```python
from build123d import *

# Parameters (mm, degrees)
F0_R      = 2
F1_DEPTH  = 100
F1_FACE_R = 2
F2_DEPTH  = 140


with BuildPart() as f1:
    # F0 (on Front) → F1 (new body)
    with BuildSketch(Plane.XZ):
        with BuildLine():
            Line((8, -2), (8, 0))
            Line((8, 0), (8, 2))
            Line((8, 2), (10, 2))
            ThreePointArc((10, 2), (10.086846, 1.501846), (10.148892, 1))
            Line((10.148892, 1), (12.459936, 1))
            ThreePointArc((12.459936, 1), (11.548494, 4.783543), (9.517612, 8.103398))
            Line((9.517612, 8.103398), (7.883457, 6.469243))
            ThreePointArc((7.883457, 6.469243), (8.194443, 6.070511), (8.485281, 5.656854))
            Line((8.485281, 5.656854), (7.071068, 4.242641))
            Line((7.071068, 4.242641), (5.656854, 5.656854))
            Line((5.656854, 5.656854), (4.242641, 7.071068))
            Line((4.242641, 7.071068), (5.656854, 8.485281))
            ThreePointArc((5.656854, 8.485281), (6.070511, 8.194443), (6.469243, 7.883457))
            Line((6.469243, 7.883457), (8.103398, 9.517612))
            ThreePointArc((8.103398, 9.517612), (4.783543, 11.548494), (1, 12.459936))
            Line((1, 12.459936), (1, 10.148892))
            ThreePointArc((1, 10.148892), (1.501846, 10.086846), (2, 10))
            Line((2, 10), (2, 8))
            Line((2, 8), (0, 8))
            Line((0, 8), (-2, 8))
            Line((-2, 8), (-2, 10))
            ThreePointArc((-2, 10), (-1.501846, 10.086846), (-1, 10.148892))
            Line((-1, 10.148892), (-1, 12.459936))
            ThreePointArc((-1, 12.459936), (-4.783543, 11.548494), (-8.103398, 9.517612))
            Line((-8.103398, 9.517612), (-6.469243, 7.883457))
            ThreePointArc((-6.469243, 7.883457), (-6.070511, 8.194443), (-5.656854, 8.485281))
            Line((-5.656854, 8.485281), (-4.242641, 7.071068))
            Line((-4.242641, 7.071068), (-5.656854, 5.656854))
            Line((-5.656854, 5.656854), (-7.071068, 4.242641))
            Line((-7.071068, 4.242641), (-8.485281, 5.656854))
            ThreePointArc((-8.485281, 5.656854), (-8.194443, 6.070511), (-7.883457, 6.469243))
            Line((-7.883457, 6.469243), (-9.517612, 8.103398))
            ThreePointArc((-9.517612, 8.103398), (-11.548494, 4.783543), (-12.459936, 1))
            Line((-12.459936, 1), (-10.148892, 1))
            ThreePointArc((-10.148892, 1), (-10.086846, 1.501846), (-10, 2))
            Line((-10, 2), (-8, 2))
            Line((-8, 2), (-8, 0))
            Line((-8, 0), (-8, -2))
            Line((-8, -2), (-10, -2))
            ThreePointArc((-10, -2), (-10.086846, -1.501846), (-10.148892, -1))
            Line((-10.148892, -1), (-12.459936, -1))
            ThreePointArc((-12.459936, -1), (-11.548494, -4.783543), (-9.517612, -8.103398))
            Line((-9.517612, -8.103398), (-7.883457, -6.469243))
            ThreePointArc((-7.883457, -6.469243), (-8.194443, -6.070511), (-8.485281, -5.656854))
            Line((-8.485281, -5.656854), (-7.071068, -4.242641))
            Line((-7.071068, -4.242641), (-5.656854, -5.656854))
            Line((-5.656854, -5.656854), (-4.242641, -7.071068))
            Line((-4.242641, -7.071068), (-5.656854, -8.485281))
            ThreePointArc((-5.656854, -8.485281), (-6.070511, -8.194443), (-6.469243, -7.883457))
            Line((-6.469243, -7.883457), (-8.103398, -9.517612))
            ThreePointArc((-8.103398, -9.517612), (-4.783543, -11.548494), (-1, -12.459936))
            Line((-1, -12.459936), (-1, -10.148892))
            ThreePointArc((-1, -10.148892), (-1.501846, -10.086846), (-2, -10))
            Line((-2, -10), (-2, -8))
            Line((-2, -8), (0, -8))
            Line((0, -8), (2, -8))
            Line((2, -8), (2, -10))
            ThreePointArc((2, -10), (1.501846, -10.086846), (1, -10.148892))
            Line((1, -10.148892), (1, -12.459936))
            ThreePointArc((1, -12.459936), (4.783543, -11.548494), (8.103398, -9.517612))
            Line((8.103398, -9.517612), (6.469243, -7.883457))
            ThreePointArc((6.469243, -7.883457), (6.070511, -8.194443), (5.656854, -8.485281))
            Line((5.656854, -8.485281), (4.242641, -7.071068))
            Line((4.242641, -7.071068), (5.656854, -5.656854))
            Line((5.656854, -5.656854), (7.071068, -4.242641))
            Line((7.071068, -4.242641), (8.485281, -5.656854))
            ThreePointArc((8.485281, -5.656854), (8.194443, -6.070511), (7.883457, -6.469243))
            Line((7.883457, -6.469243), (9.517612, -8.103398))
            ThreePointArc((9.517612, -8.103398), (11.548494, -4.783543), (12.459936, -1))
            Line((12.459936, -1), (10.148892, -1))
            ThreePointArc((10.148892, -1), (10.086846, -1.501846), (10, -2))
            Line((10, -2), (8, -2))
        make_face()
        Circle(F0_R, mode=Mode.SUBTRACT)
    extrude(amount=F1_DEPTH)

    # F1_face (on face) → F2 (join)
    with BuildSketch(Plane.XZ.offset(100)):
        with BuildLine():
            ThreePointArc((6.469243, -7.883457), (6.070511, -8.194443), (5.656854, -8.485281))
            Line((5.656854, -8.485281), (4.242641, -7.071068))
            Line((4.242641, -7.071068), (7.071068, -4.242641))
            Line((7.071068, -4.242641), (8.485281, -5.656854))
            ThreePointArc((8.485281, -5.656854), (8.194443, -6.070511), (7.883457, -6.469243))
            Line((7.883457, -6.469243), (9.517612, -8.103398))
            ThreePointArc((9.517612, -8.103398), (11.548494, -4.783543), (12.459936, -1))
            Line((12.459936, -1), (10.148892, -1))
            ThreePointArc((10.148892, -1), (10.086846, -1.501846), (10, -2))
            Line((10, -2), (8, -2))
            Line((8, -2), (8, 2))
            Line((8, 2), (10, 2))
            ThreePointArc((10, 2), (10.086846, 1.501846), (10.148892, 1))
            Line((10.148892, 1), (12.459936, 1))
            ThreePointArc((12.459936, 1), (11.548494, 4.783543), (9.517612, 8.103398))
            Line((9.517612, 8.103398), (7.883457, 6.469243))
            ThreePointArc((7.883457, 6.469243), (8.194443, 6.070511), (8.485281, 5.656854))
            Line((8.485281, 5.656854), (7.071068, 4.242641))
            Line((7.071068, 4.242641), (4.242641, 7.071068))
            Line((4.242641, 7.071068), (5.656854, 8.485281))
            ThreePointArc((5.656854, 8.485281), (6.070511, 8.194443), (6.469243, 7.883457))
            Line((6.469243, 7.883457), (8.103398, 9.517612))
            ThreePointArc((8.103398, 9.517612), (4.783543, 11.548494), (1, 12.459936))
            Line((1, 12.459936), (1, 10.148892))
            ThreePointArc((1, 10.148892), (1.501846, 10.086846), (2, 10))
            Line((2, 10), (2, 8))
            Line((2, 8), (-2, 8))
            Line((-2, 8), (-2, 10))
            ThreePointArc((-2, 10), (-1.501846, 10.086846), (-1, 10.148892))
            Line((-1, 10.148892), (-1, 12.459936))
            ThreePointArc((-1, 12.459936), (-4.783543, 11.548494), (-8.103398, 9.517612))
            Line((-8.103398, 9.517612), (-6.469243, 7.883457))
            ThreePointArc((-6.469243, 7.883457), (-6.070511, 8.194443), (-5.656854, 8.485281))
            Line((-5.656854, 8.485281), (-4.242641, 7.071068))
            Line((-4.242641, 7.071068), (-7.071068, 4.242641))
            Line((-7.071068, 4.242641), (-8.485281, 5.656854))
            ThreePointArc((-8.485281, 5.656854), (-8.194443, 6.070511), (-7.883457, 6.469243))
            Line((-7.883457, 6.469243), (-9.517612, 8.103398))
            ThreePointArc((-9.517612, 8.103398), (-11.548494, 4.783543), (-12.459936, 1))
            Line((-12.459936, 1), (-10.148892, 1))
            ThreePointArc((-10.148892, 1), (-10.086846, 1.501846), (-10, 2))
            Line((-10, 2), (-8, 2))
            Line((-8, 2), (-8, -2))
            Line((-8, -2), (-10, -2))
            ThreePointArc((-10, -2), (-10.086846, -1.501846), (-10.148892, -1))
            Line((-10.148892, -1), (-12.459936, -1))
            ThreePointArc((-12.459936, -1), (-11.548494, -4.783543), (-9.517612, -8.103398))
            Line((-9.517612, -8.103398), (-7.883457, -6.469243))
            ThreePointArc((-7.883457, -6.469243), (-8.194443, -6.070511), (-8.485281, -5.656854))
            Line((-8.485281, -5.656854), (-7.071068, -4.242641))
            Line((-7.071068, -4.242641), (-4.242641, -7.071068))
            Line((-4.242641, -7.071068), (-5.656854, -8.485281))
            ThreePointArc((-5.656854, -8.485281), (-6.070511, -8.194443), (-6.469243, -7.883457))
            Line((-6.469243, -7.883457), (-8.103398, -9.517612))
            ThreePointArc((-8.103398, -9.517612), (-4.783543, -11.548494), (-1, -12.459936))
            Line((-1, -12.459936), (-1, -10.148892))
            ThreePointArc((-1, -10.148892), (-1.501846, -10.086846), (-2, -10))
            Line((-2, -10), (-2, -8))
            Line((-2, -8), (2, -8))
            Line((2, -8), (2, -10))
            ThreePointArc((2, -10), (1.501846, -10.086846), (1, -10.148892))
            Line((1, -10.148892), (1, -12.459936))
            ThreePointArc((1, -12.459936), (4.783543, -11.548494), (8.103398, -9.517612))
            Line((8.103398, -9.517612), (6.469243, -7.883457))
        make_face()
        Circle(F1_FACE_R, mode=Mode.SUBTRACT)
    extrude(amount=F2_DEPTH)


solid = f1.part
```
For this review, take the finished solid that the model builds, in its own axes (mm). A direction names the side the tool comes from. Coordinates: 2 decimals unless noted, no trailing zeros. Put each result on its own line as item: value.
1. Mouldability with a two-part tool opening along Z and no side actions: class faces 1 (the cylindrical face through (0, -118, -2)), 2 (the flat face through (8, -118, 0)), 3 (the cylindrical face through (-11.53, -118.32, 4.83)), 4 (the cylindrical face through (4.73, -118.32, -11.57)) as released by +Z, released by -Z, zero draft, split by the parting line, or undercut.
Values found:
face 1: undercut
face 2: undercut
face 3: released by +Z
face 4: released by -Z
2. For pin 1 (0.6 mm diameter, centred on x = -9, y = -85.5, fed in from -Z); pin 2 (1.8 mm diameter, centred on y = -62.5, z = 11, fed in from +X); pin 3 (3 mm diameter, centred on x = 4, y = -87, fed in from +Z); pin 4 (2 mm diameter, centred on x = 6.5, z = 9, fed in from +Y), all flat-tipped, find the tip position at first contact; note any pin that passes through.
Values found:
pin 1: z = -7.89
pin 2: x = 7.36
pin 3: z = 12.25
pin 4: y = 0
3. Machinability: for faces 5 (the cylindrical face through (-4.83, -118.32, -11.53)), 6 (the flat face through (-8, -118, 0)), which of the approach directions +Z, -Z, +X, -X, +Y, -Y give a long, thin tool a straight path to every point of the face, cutting with its end or side? Answer none if there is none.
Values found:
face 5: -Z, -X, +Y, -Y
face 6: +Y, -Y
4. Wall thickness on probe 1 along Z at (x, y) = (0, -61.5); probe 2 along X at (y, z) = (-107, -9.5); probe 3 along X at (y, z) = (-202.5, -4.5): over which ranges is each line inside the solid? List them lowest first.
Values found:
probe 1: -8 to -2, 2 to 8
probe 2: -8.09 to -2, 2 to 8.09
probe 3: -11.66 to -7.33, -6.81 to 6.81, 7.33 to 11.66
